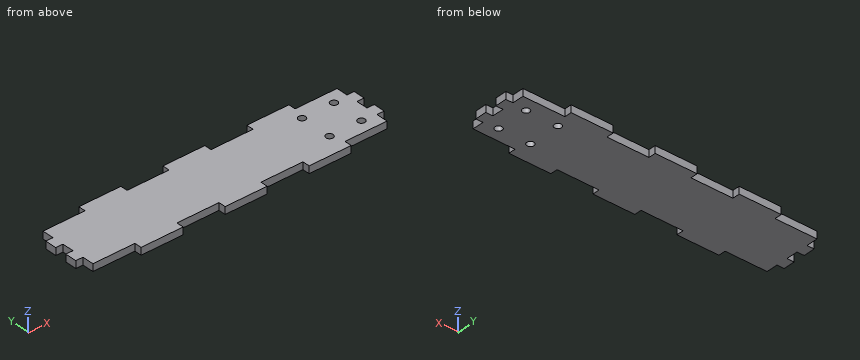
```python
from build123d import *

# Parameters (mm, degrees)
BOSS_EXTRUDE1_DEPTH = 10
SKETCH3_R           = 5
CUT_EXTRUDE1_DEPTH  = 222.151916112


with BuildPart() as part:
    # Sketch2 → Boss-Extrude1 (new body)
    with BuildSketch(Plane.XY):
        Polygon((-205.1, 40.4), (-205.1, 24.24), (-215.1, 24.24), (-215.1, 8.08), (-205.1, 8.08), (-205.1, -8.08), (-215.1, -8.08), (-215.1, -24.24), (-205.1, -24.24), (-205.1, -40.4), (-146.5, -40.4), (-146.5, -50.4), (-87.9, -50.4), (-87.9, -40.4), (-29.3, -40.4), (-29.3, -50.4), (29.3, -50.4), (29.3, -40.4), (87.9, -40.4), (87.9, -50.4), (146.5, -50.4), (146.5, -40.4), (205.1, -40.4), (205.1, -24.24), (215.1, -24.24), (215.1, -8.08), (205.1, -8.08), (205.1, 8.08), (215.1, 8.08), (215.1, 24.24), (205.1, 24.24), (205.1, 40.4), (146.5, 40.4), (146.5, 50.4), (87.9, 50.4), (87.9, 40.4), (29.3, 40.4), (29.3, 50.4), (-29.3, 50.4), (-29.3, 40.4), (-87.9, 40.4), (-87.9, 50.4), (-146.5, 50.4), (-146.5, 40.4), align=None)
    extrude(amount=BOSS_EXTRUDE1_DEPTH)

    # Sketch3 → Cut-Extrude1 (cut, through all)
    with BuildSketch(Plane.XY.offset(10)):
        with Locations((185.1, 22.225)):
            Circle(SKETCH3_R)
        with Locations((140.65, 22.225)):
            Circle(SKETCH3_R)
        with Locations((140.65, -22.225)):
            Circle(SKETCH3_R)
        with Locations((185.1, -22.225)):
            Circle(SKETCH3_R)
    extrude(amount=-CUT_EXTRUDE1_DEPTH, mode=Mode.SUBTRACT)


solid = part.part
```
For this review, take the finished solid that the model builds, in its own axes (mm). Give positions to 0.01 mm unless a question says otherwise; leave off trailing zeros. Write each loop counter-clockwise with the first axis right and the second up, starting at its lowest first coordinate (ties: lowest second). Pieces come first, ordered by that corner, then holes.
Item 1: Wall thickness on probe 1 along Y at (x, z) = (185.1, 5) (3 decimals); probe 2 along Y at (x, z) = (140.65, 2.75) (3 decimals); probe 3 along X at (y, z) = (23.5, 4): over which ranges is each line inside the solid? List them lowest first.
Item 2: Take a section at B-B (x = 140.65). Give the boundary of the cut face in (y, z) (3 decimals).
Item 3: Take a section at C-C (y = -31.5). Give the boundary of the cut face in (x, z).
Item 4: Take a section at A-A (x = 185.1). Give the boundary of the cut face in (y, z) (3 decimals), and give its area (3 significant figures).
Item 5: Take a section at D-D (z = 7.25). Give the number of separate pieces and of enclosed holes in the cut face, and give its area (3 significant figures).
Item 6: Insertion check: P1, Ø5, axis at y = 46, z = 7, coming from the +X side; P2, Ø4, axis at x = 61, z = 3.5, coming from the +Y side; P3, Ø3, axis at y = 46, z = 3.5, coming from the -X side. Each pin has a flat end and moves straight along its axis. Give the tip position at first contact, or say it passes through.
Established:
1. probe 1: y = -40.4 to -27.225, -17.225 to 17.225, 27.225 to 40.4
1. probe 2: y = -50.4 to -27.225, -17.225 to 17.225, 27.225 to 50.4
1. probe 3: x = -215.1 to 135.82, 145.48 to 180.27, 189.93 to 215.1
2. outline: (-50.4, 0) - (-27.225, 0) - (-27.225, 10) - (-50.4, 10) - close; (-17.225, 0) - (17.225, 0) - (17.225, 10) - (-17.225, 10) - close; (27.225, 0) - (50.4, 0) - (50.4, 10) - (27.225, 10) - close
3. outline: (-205.1, 0) - (205.1, 0) - (205.1, 10) - (-205.1, 10) - close
4. outline: (-40.4, 0) - (-27.225, 0) - (-27.225, 10) - (-40.4, 10) - close; (-17.225, 0) - (17.225, 0) - (17.225, 10) - (-17.225, 10) - close; (27.225, 0) - (40.4, 0) - (40.4, 10) - (27.225, 10) - close
4. area: 608 mm2
5. separate pieces: 1
5. enclosed holes: 4
5. area: 37,000 mm2
6. P1: stops at x = 146.5
6. P2: stops at y = 40.4
6. P3: stops at x = -146.5
